Here's how the part is built. I have some questions about the finished solid (model axes, mm). Give positions to 0.01 mm unless a question says otherwise; leave off trailing zeros. Loops run counter-clockwise (first coordinate to the right, second up) from the corner with the lowest first, then second, coordinate; pieces in that order, holes last.
Q1. If we section it at B-B (z = 0): Please give me the cut outline in (x, y) (3 decimals), plus the area to 3 significant figures.
Q2. Will this pin go through, and if not, where does the flat tip stop? P1, Ø1.6, axis at x = -25.4, z = 0, coming from the +Y side.
Q3. If we section it at A-A (x = 25.4): Please give me the cut outline in (y, z) (3 decimals), plus the area to 3 significant figures.
Q4. I need wall thicknesses on line 1 (Z direction, x = 25.4, y = 6.25). Which ranges of the line are inside material? Lowest first, please.
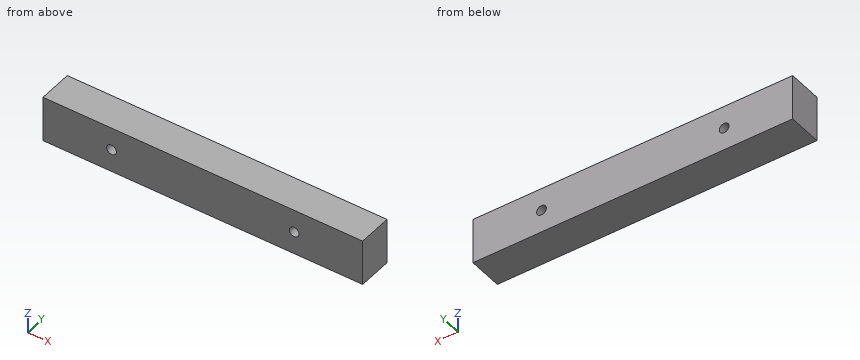
from build123d import *

# Parameters (mm, degrees)
SKETCH1_W             = 88.9
SKETCH1_H             = 12.7
BOSS_EXTRUDE1_DEPTH   = 9.525
F_6_32_TAPPED_HOLE1_D = 2.7051


with BuildPart() as part:
    # Sketch1 → Boss-Extrude1 (new body)
    with BuildSketch(Plane(origin=(0, 0, 0), x_dir=(1, 0, 0), z_dir=(0, 1, 0))):
        Rectangle(SKETCH1_W, SKETCH1_H)
    extrude(amount=BOSS_EXTRUDE1_DEPTH)

    # #6-32 Tapped Hole1 (through all)
    with Locations(Plane.XZ):
        with Locations((25.4, 0), (-25.4, 0)):
            Hole(F_6_32_TAPPED_HOLE1_D / 2)


solid = part.part
Check sheet entries:
1. outline: (-44.45, 0) - (-26.753, 0) - (-26.753, 9.525) - (-44.45, 9.525) - close; (-24.047, 0) - (24.047, 0) - (24.047, 9.525) - (-24.047, 9.525) - close; (26.753, 0) - (44.45, 0) - (44.45, 9.525) - (26.753, 9.525) - close
1. area: 795 mm2
2. P1: passes through
3. outline: (0, -6.35) - (9.525, -6.35) - (9.525, -1.353) - (0, -1.353) - close; (0, 1.353) - (9.525, 1.353) - (9.525, 6.35) - (0, 6.35) - close
3. area: 95.2 mm2
4. line 1: z = -6.35 to -1.35, 1.35 to 6.35
